Answer from the drawing. Dimensions are ordinates in mm from the lowest x, y and z of the part. A direction names the side the tool comes from. Coordinates: 2 decimals unless noted, no trailing zeros. Order: outer loops, then holes, each group sorted by start corner. A loop starts at its lowest first (then second) coordinate and runs counter-clockwise, first axis right, second up. Notation, with made-up numbers: (68, 12) - (110, 12) arc R26 ccw to (110, 37) - close; hole circle Ø5 at (-31, -4). An arc over 180 degrees is marked (long way). Use a Markdown table: item, result. Add a question column.
Item 1: For the marked faces 1 and 2, determine the directions among +Z, -Z, +X, -X, +Y, -Y from which every point of the face is accessible in a straight line to the end or side of a thin tool.
Item 2: Find the intervals of material crossed by line 1 along X through (y, z) = (5, 7.2); line 2 along Z through (x, y) = (6, 5.45); line 3 along X through (y, z) = (6, 5.75) (1 decimal), in increasing order.
Item 3: The part is cut by section A-A, the plane z = 7.2. Give the vertices of the cut face in (x, y).
Item 4: The mould has two halves that part along Z. Classify the marked faces 3, 4, 5 and 6: released by +Z, released by -Z, zero draft, split by the parting line, or undercut.
Item 5: The part is cut by section B-B, the plane y = 6. Give the vertices of the cut face in (x, z).
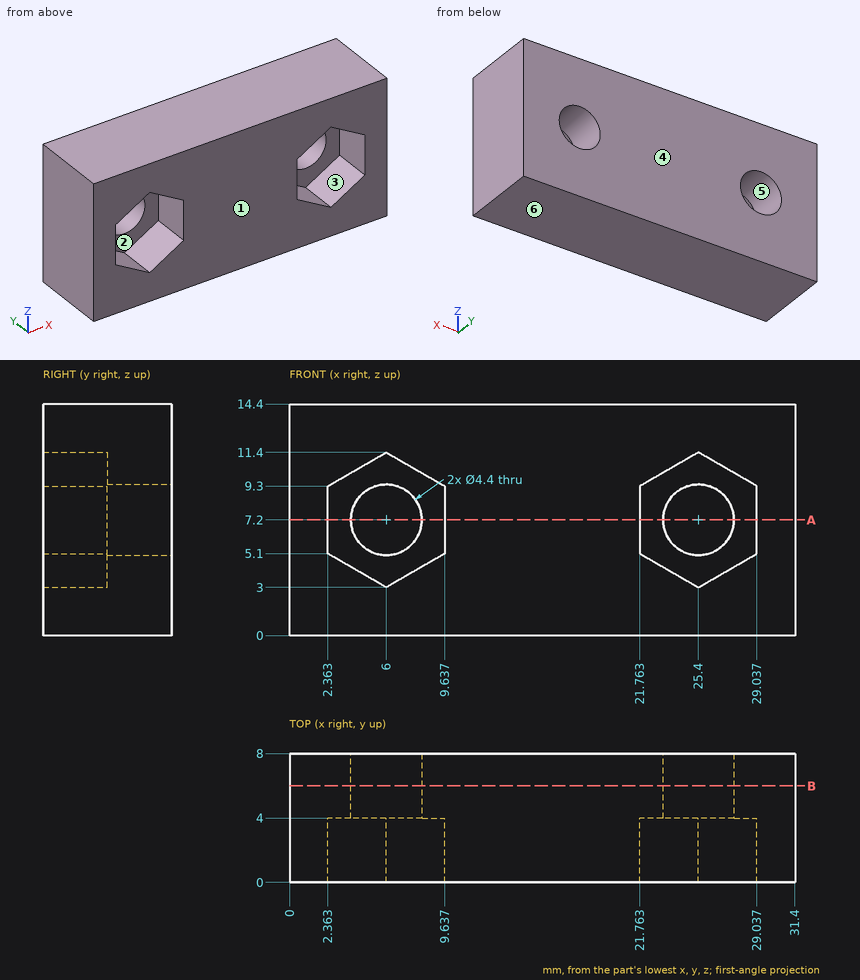
Solution:
| question | item | result |
|---|---|---|
| 1 | face 1 | +Z, -Z, +X, -X, -Y |
| 1 | face 2 | -Y |
| 2 | line 1 | x = 0 to 3.8, 8.2 to 23.2, 27.6 to 31.4 |
| 2 | line 2 | z = 0 to 5, 9.4 to 14.4 |
| 2 | line 3 | x = 0 to 4.3, 7.7 to 23.7, 27.1 to 31.4 |
| 3 | outline | (0, 0) - (2.36, 0) - (2.36, 4) - (3.8, 4) - (3.8, 8) - (0, 8) - close; (8.2, 4) - (9.64, 4) - (9.64, 0) - (21.76, 0) - (21.76, 4) - (23.2, 4) - (23.2, 8) - (8.2, 8) - close; (27.6, 4) - (29.04, 4) - (29.04, 0) - (31.4, 0) - (31.4, 8) - (27.6, 8) - close |
| 4 | face 3 | undercut |
| 4 | face 4 | zero draft |
| 4 | face 5 | undercut |
| 4 | face 6 | released by -Z |
| 5 | outline | (0, 0) - (31.4, 0) - (31.4, 14.4) - (0, 14.4) - close; hole circle Ø4.4 at (6, 7.2); hole circle Ø4.4 at (25.4, 7.2) |
